Verification items for the finished model (mm, model axes). Coordinates: 2 decimals unless noted, no trailing zeros. Order: outer loops, then holes, each group sorted by start corner. A loop starts at its lowest first (then second) coordinate and runs counter-clockwise, first axis right, second up. Notation, with made-up numbers: M 66.25,75.25 L 107.25,75.25 A34 cw 107.25,114.25 Z; hole C -13.5,72 d2. An arc over 180 degrees is marked long. Write item = value, one per line.
```python
from build123d import *

# Parameters (mm, degrees)
SKETCH1_W                    = 6.35
SKETCH1_H                    = 127
BOSS_EXTRUDE1_DEPTH          = 25.4
M2_5X0_45_TAPPED_HOLE1_D     = 2.05
M2_5X0_45_TAPPED_HOLE1_DEPTH = 6.35
M2_5X0_45_TAPPED_HOLE1_TIP   = 0.615882135
CUT_EXTRUDE1_DEPTH           = 69.685751798
CUT_EXTRUDE1_DEPTH_BACK      = 69.685751798


with BuildPart() as part:
    # Sketch1 → Boss-Extrude1 (new body)
    with BuildSketch(Plane(origin=(0, 0, 0), x_dir=(0, 0, -1), z_dir=(1, 0, 0))):
        Rectangle(SKETCH1_W, SKETCH1_H)
    extrude(amount=BOSS_EXTRUDE1_DEPTH)

    # M2.5x0.45 Tapped Hole1
    with Locations(Plane.ZY):
        with Locations((0, 53.5), (0, 26.75), (0, 0), (0, -26.75), (0, -53.5)):
            Hole(M2_5X0_45_TAPPED_HOLE1_D / 2, depth=M2_5X0_45_TAPPED_HOLE1_DEPTH)
            with Locations((0, 0, -(M2_5X0_45_TAPPED_HOLE1_DEPTH + M2_5X0_45_TAPPED_HOLE1_TIP / 2))):  # 118° drill point
                Cone(0, M2_5X0_45_TAPPED_HOLE1_D / 2, M2_5X0_45_TAPPED_HOLE1_TIP, mode=Mode.SUBTRACT)

    # Sketch4 → Cut-Extrude1 (cut, two sides: drawn at the far end of the back side and taken through both)
    with BuildSketch(Plane.XY.offset(3.175).offset(-CUT_EXTRUDE1_DEPTH_BACK)):
        Polygon((25.4, 63.5), (12.7, 63.5), (25.4, 0), align=None)
    extrude(amount=CUT_EXTRUDE1_DEPTH + CUT_EXTRUDE1_DEPTH_BACK, mode=Mode.SUBTRACT)


solid = part.part
```
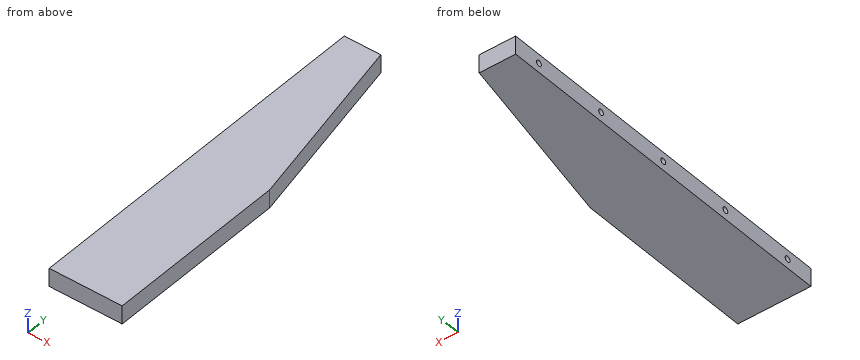
Item 1: Sectioned sample at C-C, the plane x = 19.25. Enter the section's corners in (y, z) (3 decimals), then the cut area to 3 significant figures.
Report:
outline = M -63.5,-3.175 L 30.75,-3.175 L 30.75,3.175 L -63.5,3.175 Z
area = 598 mm^2
Item 2: Scan lines: L1, parallel to Y at x = 2.75, z = 0 (3 decimals); L2, parallel to Z at x = 2.5, y = 0 (3 decimals); L3, parallel to Z at x = 2.75, y = -53 (3 decimals). Record each from-to range of solid material in increasing order. Write a range as from..to.
Report:
L1 = -63.5..-54.525, -52.475..-27.775, -25.725..-1.025, 1.025..25.725, 27.775..52.475, 54.525..63.5
L2 = -3.175..-1.025, 1.025..3.175
L3 = -3.175..-0.895, 0.895..3.175
Item 3: Gauge pin test, flat end, axial feed: pin 1 (1.6 mm diameter, centred on y = 53.5, z = 0, fed in from +X). Record the tip position at first contact, or that the pin passes through.
Report:
pin_1 = 14.86
Item 4: Sectioned sample at B-B, the plane z = -2. Enter the section's corners in (x, y).
Report:
outline = M 0,-63.5 L 25.4,-63.5 L 25.4,0 L 12.7,63.5 L 0,63.5 Z
Item 5: Sectioned sample at A-A, the plane x = 5. Enter the section's corners in (y, z) (3 decimals), then the cut area to 3 significant figures.
Report:
outline = M -63.5,-3.175 L 63.5,-3.175 L 63.5,3.175 L -63.5,3.175 Z; hole C -53.5,0 d2.05; hole C -26.75,0 d2.05; hole C 0,0 d2.05; hole C 26.75,0 d2.05; hole C 53.5,0 d2.05
area = 790 mm^2
